Work out the finished part from the listing and answer in its coordinate system (mm). A direction names the side the tool comes from. Round coordinates to 2 decimals unless told otherwise and drop trailing zeros. Order: outer loops, then holes, each group sorted by start corner. A loop starts at its lowest first (then second) coordinate and runs counter-clockwise, first axis right, second up.
from build123d import *

# Parameters (mm, degrees)
F1_DEPTH = 80
F2_W     = 40
F2_H     = 26
F3_DEPTH = 20


with BuildPart() as f1:
    # F0 (on Front) → F1 (new body)
    with BuildSketch(Plane.XZ):
        Polygon((-82.429772, -14.864372), (57.570228, -14.864372), (57.570228, 11.135628), (-1.449937, 11.135628), (-1.449937, 37.135628), (-22.429772, 37.135628), (-22.429772, 63.135628), (-37.429772, 63.135628), (-52.429772, 49.906872), (-67.429772, 63.135628), (-82.429772, 63.135628), align=None)
    extrude(amount=F1_DEPTH)

    # F2 (on face) → F3 (cut)
    with BuildSketch(Plane.YZ.offset(57.570228)):
        with Locations((-40, -1.864372)):
            Rectangle(F2_W, F2_H)
    extrude(amount=-F3_DEPTH, mode=Mode.SUBTRACT)


solid = f1.part
Item 1: Find section C-C (z = 53.5). Write down the section's boundary in (x, y).
Item 2: For a pull along X with two mould halves and no side action, classify faces 5 (the face through (48, -60, -2)), 6 (the face through (37.57, -40, -2)), 7 (the face through (-44.825, -39.44, 56.614)) as released by +X, released by -X, zero draft, split by the parting line, or undercut.
Item 3: Given pin 1 (10.5 mm diameter, centred on x = -16.5, y = -56, fed in from +Z); pin 2 (10 mm diameter, centred on y = -13, z = 39, fed in from +X); pin 3 (4 mm diameter, centred on y = -71, z = 44.5, fed in from +X), each flat-ended and moving along its own axis, determine where each tip first touches the part or whether it passes through.
Item 4: Find section A-A (x = 39.5). Write down the section's boundary in (y, z).
Item 5: Find section D-D (z = 6). Write down the section's boundary in (x, y), plus the area to 3 significant figures.
Item 6: A tool of negligible diameter and unlimited length cuts with its end or side. For faces 1 (the face through (-22.43, -39, 50)), 2 (the face through (48, -20, -2)), 3 (the face through (-59.825, -39.44, 56.429)), 4 (the face through (-82.43, -39, 25)), from which of +Z, -Z, +X, -X, +Y, -Y can it reach the whole face along a straight path? Write none if from no direction.
Item 7: Find section B-B (y = -41.5). Write down the section's boundary in (x, z).
Item 8: Find the intervals of material crossed by line 1 along Y through (x, z) = (43, 4.5); line 2 along X through (y, z) = (-47, 30.5); line 3 along Z through (x, y) = (29, -5), in increasing order.
Model answer:
1. outline: (-82.43, -80) - (-56.5, -80) - (-56.5, 0) - (-82.43, 0) - close; (-48.36, -80) - (-22.43, -80) - (-22.43, 0) - (-48.36, 0) - close
2. face 5: zero draft
2. face 6: released by +X
2. face 7: undercut
3. pin 1: stops at z = 37.14
3. pin 2: stops at x = -1.45
3. pin 3: stops at x = -22.43
4. outline: (-80, -14.86) - (-60, -14.86) - (-60, 11.14) - (-80, 11.14) - close; (-20, -14.86) - (0, -14.86) - (0, 11.14) - (-20, 11.14) - close
5. outline: (-82.43, -80) - (57.57, -80) - (57.57, -60) - (37.57, -60) - (37.57, -20) - (57.57, -20) - (57.57, 0) - (-82.43, 0) - close
5. area: 10,400 mm2
6. face 1: +Z, +X, +Y, -Y
6. face 2: +Z, -Z, +X
6. face 3: +Z, +Y, -Y
6. face 4: +Z, -Z, -X, +Y, -Y
7. outline: (-82.43, -14.86) - (37.57, -14.86) - (37.57, 11.14) - (-1.45, 11.14) - (-1.45, 37.14) - (-22.43, 37.14) - (-22.43, 63.14) - (-37.43, 63.14) - (-52.43, 49.91) - (-67.43, 63.14) - (-82.43, 63.14) - close
8. line 1: y = -80 to -60, -20 to 0
8. line 2: x = -82.43 to -1.45
8. line 3: z = -14.86 to 11.14
